Read the model definition and answer for the solid it produces. Units are mm, in the model's axes. Face numbers are marked on the shaded views. A direction names the side the tool comes from. Coordinates: 2 decimals unless noted, no trailing zeros. Loops run counter-clockwise (first coordinate to the right, second up) from the corner with the lowest first, then second, coordinate; pieces in that order, holes last.
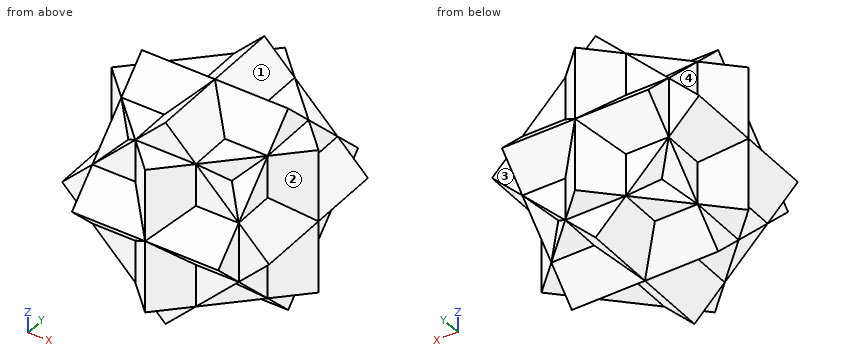
from build123d import *

# Parameters (mm, degrees)
F1_DEPTH = 25
F3_DEPTH = 25
F5_DEPTH = 25


with BuildPart() as f1:
    # F0 (on Front) → F1 (new body, symmetric)
    with BuildSketch(Plane.XZ):
        Polygon((35.355339, 0), (0, 35.355339), (-35.355339, 0), (0, -35.355339), align=None)
    extrude(amount=F1_DEPTH, both=True)

    # F2 (on Right) → F3 (join, symmetric)
    with BuildSketch(Plane.YZ):
        Polygon((35.355339, 0), (0, 35.355339), (-35.355339, 0), (0, -35.355339), align=None)
    extrude(amount=F3_DEPTH, both=True)

    # F4 (on Top) → F5 (join, symmetric)
    with BuildSketch(Plane.XY):
        Polygon((-35.355339, 0), (0, -35.355339), (35.355339, 0), (0, 35.355339), align=None)
    extrude(amount=F5_DEPTH, both=True)


solid = f1.part
Q1. A cutting plane is placed at C-C (x = 14.5). Give the vertices of the cut face in (y, z).
Findings below:
outline: (-35.36, 0) - (-25, -10.36) - (-25, -20.86) - (-20.86, -20.86) - (-20.86, -25) - (-10.36, -25) - (0, -35.36) - (10.36, -25) - (20.86, -25) - (20.86, -20.86) - (25, -20.86) - (25, -10.36) - (35.36, 0) - (25, 10.36) - (25, 20.86) - (20.86, 20.86) - (20.86, 25) - (10.36, 25) - (0, 35.36) - (-10.36, 25) - (-20.86, 25) - (-20.86, 20.86) - (-25, 20.86) - (-25, 10.36) - close
Q2. Which of the six approach directions +Z, -Z, +X, -X, +Y, -Y give full straight-line access (tool end or side, diameter ignored) to the marked faces 1, 2, 3 and 4?
Findings below:
face 1: +Z, +X, +Y
face 2: +Z, +X, -Y
face 3: +Z, -Z, +X, +Y
face 4: +Z, -X, +Y
Q3. Flat-ended cylindrical pins translate along their axes: pin 1 Ø1 at (x, z) = (-22, -14) entering from -Y; pin 2 Ø11.5 at (x, z) = (-18.5, -20) entering from +Y; pin 3 Ø1.5 at (y, z) = (-3, 16) entering from +X. Find the tip coordinate at first contact, or state that the pin passes through.
Findings below:
pin 1: stops at y = -25
pin 2: stops at y = 25
pin 3: stops at x = 33.11
Q4. A cutting plane is placed at D-D (z = -8). Give the vertices of the cut face in (x, y).
Findings below:
outline: (-35.36, 0) - (-27.36, -8) - (-27.36, -25) - (-25, -25) - (-25, -27.36) - (-8, -27.36) - (0, -35.36) - (8, -27.36) - (25, -27.36) - (25, -25) - (27.36, -25) - (27.36, -8) - (35.36, 0) - (27.36, 8) - (27.36, 25) - (25, 25) - (25, 27.36) - (8, 27.36) - (0, 35.36) - (-8, 27.36) - (-25, 27.36) - (-25, 25) - (-27.36, 25) - (-27.36, 8) - close
Q5. A cutting plane is placed at B-B (z = 27). Give the vertices of the cut face in (x, y), then the cut area to 3 significant figures.
Findings below:
outline: (-25, -8.36) - (-8.36, -8.36) - (-8.36, -25) - (8.36, -25) - (8.36, -8.36) - (25, -8.36) - (25, 8.36) - (8.36, 8.36) - (8.36, 25) - (-8.36, 25) - (-8.36, 8.36) - (-25, 8.36) - close
area: 1,390 mm2
Q6. A cutting plane is placed at A-A (y = -19.5). Give the vertices of the cut face in (x, z), then the cut area to 3 significant figures.
Findings below:
outline: (-35.36, 0) - (-25, -10.36) - (-25, -15.86) - (-19.5, -15.86) - (-15.86, -19.5) - (-15.86, -25) - (-10.36, -25) - (0, -35.36) - (10.36, -25) - (15.86, -25) - (15.86, -19.5) - (19.5, -15.86) - (25, -15.86) - (25, -10.36) - (35.36, 0) - (25, 10.36) - (25, 15.86) - (19.5, 15.86) - (15.86, 19.5) - (15.86, 25) - (10.36, 25) - (0, 35.36) - (-10.36, 25) - (-15.86, 25) - (-15.86, 19.5) - (-19.5, 15.86) - (-25, 15.86) - (-25, 10.36) - close
area: 2,620 mm2
Q7. A straight line is drawn through the part: probe 1 along X at (y, z) = (19, -14). Find the intervals that lie inside material, in ascending order.
Findings below:
probe 1: x = -25 to 25
